The drawing under review shows one solid part. Ordinate dimensions are in mm from its lowest x, y, z. Coordinates: 2 decimals unless noted, no trailing zeros. Write each loop counter-clockwise with the first axis right and the second up, starting at its lowest first coordinate (ties: lowest second). Pieces come first, ordered by that corner, then holes.
Q1. For probe 1 along X at (y, z) = (2.5, 9.75); probe 2 along Z at (x, y) = (15, 3.85); probe 3 along Y at (x, z) = (5, 23), list the stretches that pass through material, from the lowest coordinate up.
Q2. Take a section at B-B (z = 11). Give the boundary of the cut face in (x, y), and give its area (3 significant figures).
Q3. Take a section at C-C (z = 15). Give the boundary of the cut face in (x, y).
Q4. Take a section at D-D (y = 2.5). Give the boundary of the cut face in (x, z), and give its area (3 significant figures).
Q5. Mouldability with a two-part tool opening along Z and no side actions: class the marked faces 1, 2 and 3 as pulls with the +Z half, pulls with the -Z half, needs draft (parallel to the pull), parting line crosses it, or undercut.
Q6. Take a section at A-A (x = 15). Give the boundary of the cut face in (y, z), and give its area (3 significant figures).
Q7. Insertion check: pin 1 (2 mm diameter, centred on x = 20, y = 2.5, fed in from -Z). The pin has a flat end and moves straight along its axis. Give the tip position at first contact, or say it passes through.
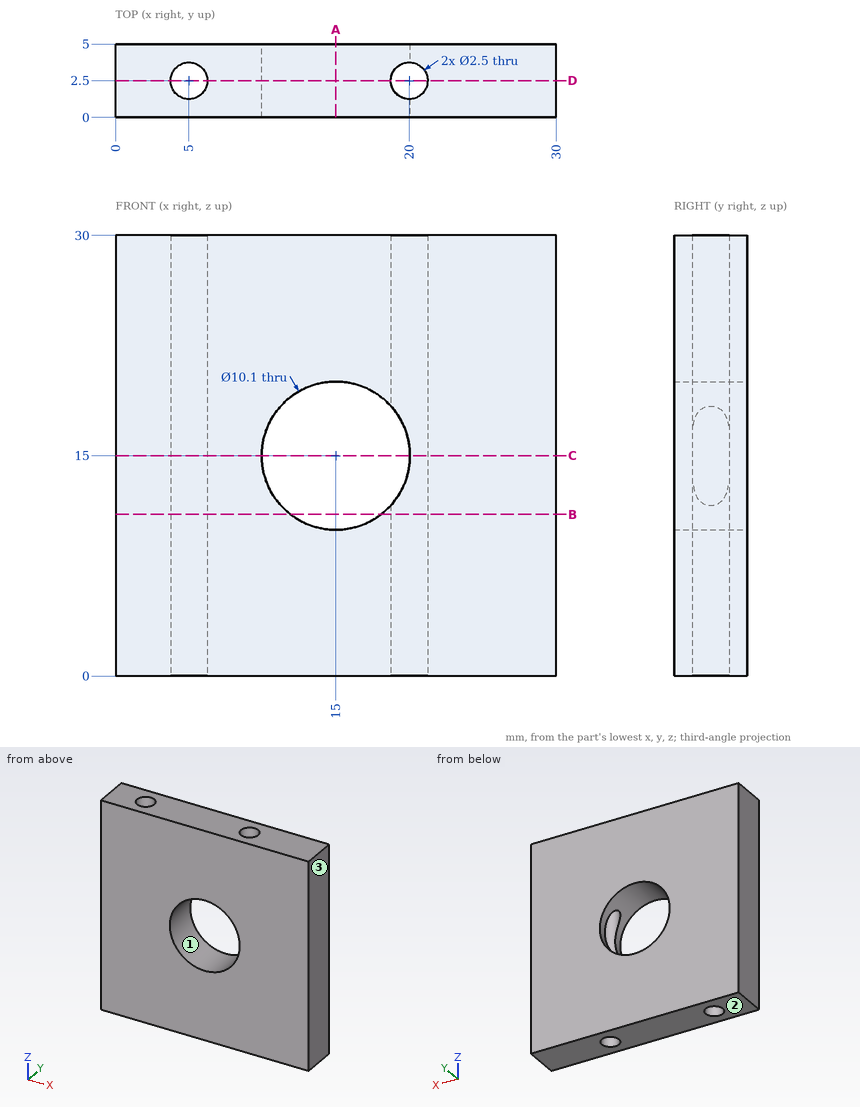
Response:
1. probe 1: x = 0 to 3.75, 6.25 to 18.75, 21.25 to 30
1. probe 2: z = 0 to 9.95, 20.05 to 30
1. probe 3: y = 0 to 1.25, 3.75 to 5
2. outline: (0, 0) - (11.92, 0) - (11.92, 5) - (0, 5) - close; (18.08, 0) - (30, 0) - (30, 5) - (18.08, 5) - close; hole circle Ø2.5 at (5, 2.5); hole circle Ø2.5 at (20, 2.5)
2. area: 109 mm2
3. outline: (0, 0) - (9.95, 0) - (9.95, 5) - (0, 5) - close; (20.05, 0) - (30, 0) - (30, 5) - (20.05, 5) - (20.05, 3.75) arc R1.25 cw to (20.05, 1.25) - close; hole circle Ø2.5 at (5, 2.5)
4. outline: (0, 0) - (3.75, 0) - (3.75, 30) - (0, 30) - close; (6.25, 0) - (18.75, 0) - (18.75, 11.62) arc R5.05 cw (long way) to (18.75, 18.38) - (18.75, 30) - (6.25, 30) - close; (21.25, 0) - (30, 0) - (30, 30) - (21.25, 30) - close
4. area: 676 mm2
5. face 1: undercut
5. face 2: pulls with the -Z half
5. face 3: needs draft
6. outline: (0, 0) - (5, 0) - (5, 9.95) - (0, 9.95) - close; (0, 20.05) - (5, 20.05) - (5, 30) - (0, 30) - close
6. area: 99.5 mm2
7. pin 1: passes through
